```python
from build123d import *

# Parameters (mm, degrees)
F0_R      = 23.25
F0_R_2    = 5
F1_DEPTH  = 1
F2_R      = 25
F2_R_2    = 23.25
F2_R_3    = 5
F3_DEPTH  = 1.2
F4_R      = 27
F4_R_2    = 25
F4_R_3    = 5
F5_DEPTH  = 6
F6_R      = 22
F6_R_2    = 5
F7_DEPTH  = 6
F8_R      = 25
F8_R_2    = 22
F9_DEPTH  = 5
F10_R     = 21
F10_R_2   = 5
F11_DEPTH = 0.5


with BuildPart() as f1:
    # F0 (on Top) → F1 (new body)
    with BuildSketch(Plane.XY):
        Circle(F0_R)
        Circle(F0_R_2, mode=Mode.SUBTRACT)
    extrude(amount=F1_DEPTH)

    # F2 (on face) → F3 (join)
    with BuildSketch(Plane.XY.offset(1)):
        Circle(F2_R)
        Circle(F2_R_2, mode=Mode.SUBTRACT)
        Circle(F2_R_2)
        Circle(F2_R_3, mode=Mode.SUBTRACT)
    extrude(amount=F3_DEPTH)

    # F4 (on face) → F5 (join)
    with BuildSketch(Plane.XY.offset(2.2)):
        Circle(F4_R)
        Circle(F4_R_2, mode=Mode.SUBTRACT)
        Circle(F4_R_2)
        Circle(F4_R_3, mode=Mode.SUBTRACT)
    extrude(amount=F5_DEPTH)

    # F6 (on face) → F7 (cut)
    with BuildSketch(Plane.XY.offset(8.2)):
        Circle(F6_R)
        Circle(F6_R_2, mode=Mode.SUBTRACT)
    extrude(amount=-F7_DEPTH, mode=Mode.SUBTRACT)

    # F8 (on face) → F9 (cut)
    with BuildSketch(Plane.XY.offset(8.2)):
        Circle(F8_R)
        Circle(F8_R_2, mode=Mode.SUBTRACT)
    extrude(amount=-F9_DEPTH, mode=Mode.SUBTRACT)

    # F10 (on face) → F11 (cut)
    with BuildSketch(Plane(origin=(0, 0, 0), x_dir=(1, 0, 0), z_dir=(0, 0, -1))):
        Circle(F10_R)
        Circle(F10_R_2, mode=Mode.SUBTRACT)
    extrude(amount=-F11_DEPTH, mode=Mode.SUBTRACT)


solid = f1.part
```
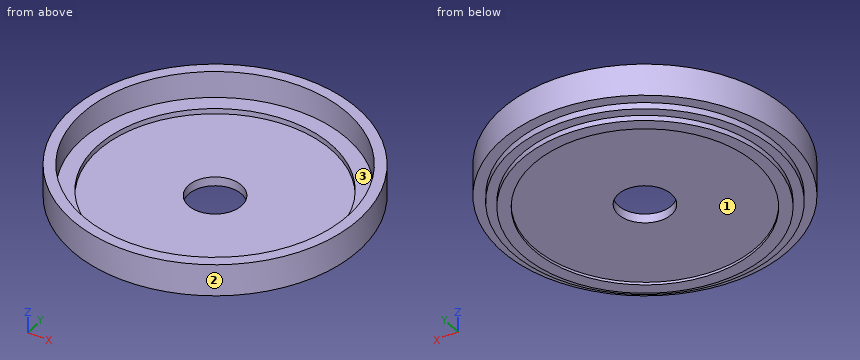
For this review, take the finished solid that the model builds, in its own axes (mm). Face numbers are marked on the shaded views. Coordinates: 2 decimals unless noted, no trailing zeros. Write each loop counter-clockwise with the first axis right and the second up, starting at its lowest first coordinate (ties: lowest second). Pieces come first, ordered by that corner, then holes. Notation, with made-up numbers: (-12.75, 3.5) - (33.25, 3.5) arc R31 cw to (33.25, 36.5) - close; hole circle Ø2 at (-6.75, 24.25). An arc over 180 degrees is marked (long way). Put each result on its own line as item: value.
1. Add section A-A, the plane x = 0. Give the boundary of the cut face in (y, z).
Values found:
outline: (-27, 2.2) - (-25, 2.2) - (-25, 1) - (-23.25, 1) - (-23.25, 0) - (-21, 0) - (-21, 0.5) - (-5, 0.5) - (-5, 2.2) - (-22, 2.2) - (-22, 3.2) - (-25, 3.2) - (-25, 8.2) - (-27, 8.2) - close; (5, 0.5) - (21, 0.5) - (21, 0) - (23.25, 0) - (23.25, 1) - (25, 1) - (25, 2.2) - (27, 2.2) - (27, 8.2) - (25, 8.2) - (25, 3.2) - (22, 3.2) - (22, 2.2) - (5, 2.2) - close
2. Mouldability with a two-part tool opening along Y and no side actions: class the marked faces 1, 2 and 3 as released by +Y, released by -Y, zero draft, split by the parting line, or undercut.
Values found:
face 1: undercut
face 2: split by the parting line
face 3: undercut
3. Wall thickness on probe 1 along Y at (x, z) = (0, 0.2); probe 2 along Y at (x, z) = (0, 0.9); probe 3 along Z at (x, y) = (-9, -6): over which ranges is each line inside the solid? List them lowest first.
Values found:
probe 1: -23.25 to -21, 21 to 23.25
probe 2: -23.25 to -5, 5 to 23.25
probe 3: 0.5 to 2.2
4. Add section C-C, the plane x = 8.5. Give the boundary of the cut face in (y, z), then the cut area to 3 significant figures.
Values found:
outline: (-25.63, 2.2) - (-23.51, 2.2) - (-23.51, 1) - (-21.64, 1) - (-21.64, 0) - (-19.2, 0) - (-19.2, 0.5) - (19.2, 0.5) - (19.2, 0) - (21.64, 0) - (21.64, 1) - (23.51, 1) - (23.51, 2.2) - (25.63, 2.2) - (25.63, 8.2) - (23.51, 8.2) - (23.51, 3.2) - (20.29, 3.2) - (20.29, 2.2) - (-20.29, 2.2) - (-20.29, 3.2) - (-23.51, 3.2) - (-23.51, 8.2) - (-25.63, 8.2) - close
area: 112 mm²
5. For pin 1 (6 mm diameter, centred on x = 4, y = -16.5, fed in from -Z); pin 2 (16 mm diameter, centred on x = -11, y = 7, fed in from -Z); pin 3 (1 mm diameter, centred on x = 7.5, y = 6.5, fed in from +Z); pin 4 (4 mm diameter, centred on y = 3.5, z = 3, fed in from +X), all flat-tipped, find the tip position at first contact; note any pin that passes through.
Values found:
pin 1: z = 0.5
pin 2: z = 0
pin 3: z = 2.2
pin 4: x = 26.96
